```python
from build123d import *

# Parameters (mm, degrees)
SKIZZE2_2_W                     = 38
SKIZZE2_2_H                     = 48.5
AUFSATZ_LINEAR_AUSTRAGEN1_DEPTH = 2
SKIZZE4_R                       = 2.5
SKIZZE4_R_2                     = 1.5
AUFSATZ_LINEAR_AUSTRAGEN2_DEPTH = 3
SKIZZE5_R                       = 0.4
SKIZZE5_R_2                     = 0.9
SKIZZE5_R_3                     = 1.4
AUFSATZ_LINEAR_AUSTRAGEN3_DEPTH = 3


with BuildPart() as part:
    # Skizze1 → Ausformung3 section 0
    with BuildSketch(Plane(origin=(0, 0, 0), x_dir=(0, 1, 0), z_dir=(0, 0, 1))):
        with BuildLine():
            Line((0, 9.7), (-8.400446417, 4.85))
            Line((-8.400446417, 4.85), (-8.400446417, -4.85))
            Line((-8.400446417, -4.85), (0, -9.7))
            Line((0, -9.7), (8.400446417, -4.85))
            Line((8.400446417, -4.85), (8.400446417, 4.85))
            Line((8.400446417, 4.85), (0, 9.7))
        make_face()
    # Skizze3 → Ausformung3 section 1
    with BuildSketch(Plane(origin=(0, 0, 2.5), x_dir=(0, 1, 0), z_dir=(0, 0, 1))):
        with BuildLine():
            Line((8.400446417, 4.85), (0, 9.7))
            Line((0, 9.7), (-8.400446417, 4.85))
            Line((-8.400446417, 4.85), (-8.400446417, -4.85))
            Line((-8.400446417, -4.85), (0, -9.7))
            Line((0, -9.7), (8.400446417, -4.85))
            Line((8.400446417, -4.85), (8.400446417, 4.85))
        make_face()
    loft()

    # Ausformung4: read off the stored shape, not the designer's step
    # Ausformung4: loft between two sections, ruled curve by curve
    ausformung4_from = [
        Edge.make_bspline([(24.25, 19, 5), (24.25, 12.666666667, 5), (24.25, 6.333333333, 5), (24.25, -6.333333333, 5), (24.25, -12.666666667, 5), (24.25, -19, 5)], [0, 0, 0, 0, 0.5, 0.5, 1, 1, 1, 1], 3),
        Edge.make_bspline([(0, -19, 5), (-4.041666667, -19, 5), (-8.083333333, -19, 5), (-16.166666667, -19, 5), (-20.208333333, -19, 5), (-24.25, -19, 5)], [0, 0, 0, 0, 0.5, 0.5, 1, 1, 1, 1], 3),
        Edge.make_bspline([(-24.25, -19, 5), (-24.25, -12.666666667, 5), (-24.25, -6.333333333, 5), (-24.25, 6.333333333, 5), (-24.25, 12.666666667, 5), (-24.25, 19, 5)], [0, 0, 0, 0, 0.5, 0.5, 1, 1, 1, 1], 3),
        Edge.make_bspline([(0, 19, 5), (4.041666667, 19, 5), (8.083333333, 19, 5), (16.166666667, 19, 5), (20.208333333, 19, 5), (24.25, 19, 5)], [0, 0, 0, 0, 0.5, 0.5, 1, 1, 1, 1], 3),
        Edge.make_line((0, -19, 5), (24.25, -19, 5)),
        Edge.make_line((0, 19, 5), (-24.25, 19, 5)),
    ]
    ausformung4_to = [
        Edge.make_bspline([(9.7, 0, 2.5), (8.891666667, -1.400074403, 2.5), (8.083333333, -2.800148806, 2.5), (6.466666667, -5.600297611, 2.5), (5.658333333, -7.000372014, 2.5), (4.85, -8.400446417, 2.5)], [0, 0, 0, 0, 0.5, 0.5, 1, 1, 1, 1], 3),
        Edge.make_bspline([(-4.85, -8.400446417, 2.5), (-5.658333333, -7.000372014, 2.5), (-6.466666667, -5.600297611, 2.5), (-8.083333333, -2.800148806, 2.5), (-8.891666667, -1.400074403, 2.5), (-9.7, 0, 2.5)], [0, 0, 0, 0, 0.5, 0.5, 1, 1, 1, 1], 3),
        Edge.make_bspline([(-9.7, 0, 2.5), (-8.891666667, 1.400074403, 2.5), (-8.083333333, 2.800148806, 2.5), (-6.466666667, 5.600297611, 2.5), (-5.658333333, 7.000372014, 2.5), (-4.85, 8.400446417, 2.5)], [0, 0, 0, 0, 0.5, 0.5, 1, 1, 1, 1], 3),
        Edge.make_bspline([(4.85, 8.400446417, 2.5), (5.658333333, 7.000372014, 2.5), (6.466666667, 5.600297611, 2.5), (8.083333333, 2.800148806, 2.5), (8.891666667, 1.400074403, 2.5), (9.7, 0, 2.5)], [0, 0, 0, 0, 0.5, 0.5, 1, 1, 1, 1], 3),
        Edge.make_line((-4.85, -8.400446417, 2.5), (4.85, -8.400446417, 2.5)),
        Edge.make_line((4.85, 8.400446417, 2.5), (-4.85, 8.400446417, 2.5)),
    ]
    ausformung4 = Solid(Shell([*[Face.make_surface_from_curves(ausformung4_from[k], ausformung4_to[k]) for k in range(6)], Face(Wire(ausformung4_from)), Face(Wire(ausformung4_to))]))
    add(ausformung4)

    # Skizze2<2> → Aufsatz-Linear austragen1 (add)
    with BuildSketch(Plane(origin=(0, 0, 5), x_dir=(0, 1, 0), z_dir=(0, 0, 1))):
        Rectangle(SKIZZE2_2_W, SKIZZE2_2_H)
    extrude(amount=AUFSATZ_LINEAR_AUSTRAGEN1_DEPTH)

    # Skizze4 → Aufsatz-Linear austragen2 (add)
    with BuildSketch(Plane.XY.offset(7)):
        with Locations((-20.75, 0)):
            Circle(SKIZZE4_R)
        with Locations((20.75, 0)):
            Circle(SKIZZE4_R)
        with Locations(Location((-22.75, 16, 0), (0, 0, 180))):
            Circle(SKIZZE4_R_2)
        with Locations(Location((-22.75, -16, 0), (0, 0, 180))):
            Circle(SKIZZE4_R_2)
        with Locations((22.25, 16)):
            Circle(SKIZZE4_R_2)
        with Locations((22.25, -16)):
            Circle(SKIZZE4_R_2)
    extrude(amount=AUFSATZ_LINEAR_AUSTRAGEN2_DEPTH)

    # Skizze5 → Aufsatz-Linear austragen3 (add)
    with BuildSketch(Plane.XY.offset(10)):
        with Locations((-22.75, 16)):
            Circle(SKIZZE5_R)
        with Locations((-22.75, -16)):
            Circle(SKIZZE5_R_2)
        with Locations((-20.75, 0)):
            Circle(SKIZZE5_R_3)
        with Locations((20.75, 0)):
            Circle(SKIZZE5_R_3)
        with Locations((22.25, 16)):
            Circle(SKIZZE5_R_2)
        with Locations((22.25, -16)):
            Circle(SKIZZE5_R_2)
    extrude(amount=AUFSATZ_LINEAR_AUSTRAGEN3_DEPTH)


solid = part.part
```
Build history of the part. All positions in model axes, mm. A direction names the side the tool comes from. Give positions to 0.01 mm unless a question says otherwise; leave off trailing zeros. Loops run counter-clockwise (first coordinate to the right, second up) from the corner with the lowest first, then second, coordinate; pieces in that order, holes last.
1) 3-axis set-ups, long thin cutter, end or side, ignore diameter. For faces 1 (the face through (0, -8.4, 1)), 2 (the face through (-23, -16, 13)), 3 (the face through (7.24, -4.26, 1.27)), 4 (the face through (0, 8.4, 1)), 5 (the face through (-21.25, 15.93, 8.48)): which of +Z, -Z, +X, -X, +Y, -Y reach the whole face in a straight line?
Values follow:
face 1: -Z, +X, -X, -Y
face 2: +Z, +X, -X, +Y, -Y
face 3: -Z, +X, -Y
face 4: -Z, +X, -X, +Y
face 5: +Z
2) Two-plate mould, pull along Y, no slides. Class faces 6 (the face through (22, -1, 10)), 7 (the face through (-7.24, 4.26, 1.27)), 8 (the face through (-7.31, -4.14, 1.27)): released by +Y, released by -Y, zero draft, split by the parting line, or undercut.
Values follow:
face 6: undercut
face 7: released by +Y
face 8: released by -Y
3) Drop flat-ended pins along their axis: P1, Ø4, axis at x = 10, y = -11, coming from the -Z side; P2, Ø2.5, axis at x = -23, y = 15.5, coming from the +Z side; P3, Ø19, axis at x = -2, y = 9, coming from the +Z side; P4, Ø3, axis at y = 3, z = 10, coming from the -X side. Give the stop position or say it passes through.
Values follow:
P1: stops at z = 2.93
P2: stops at z = 13
P3: stops at z = 7
P4: stops at x = -22.75
4) Band-saw the part on A-A on z = 11. List the corners of the cut face in (x, y).
Values follow:
outline: circle Ø1.8 at (-22.75, -16); circle Ø0.8 at (-22.75, 16); circle Ø2.8 at (-20.75, 0); circle Ø2.8 at (20.75, 0); circle Ø1.8 at (22.25, -16); circle Ø1.8 at (22.25, 16)
5) Probe line 1 along Z through (x, y) = (5, 7); line 2 along X through (y, z) = (15.5, 8); line 3 along Z through (x, y) = (4.5, -11). List the from-to ranges inside material, lowest first.
Values follow:
line 1: z = 0 to 7
line 2: x = -24.16 to -21.34, 20.84 to 23.66
line 3: z = 3.11 to 7
